Work out the finished part from the listing and answer in its coordinate system (mm). A direction names the side the tool comes from. Round coordinates to 2 decimals unless told otherwise and drop trailing zeros. Order: outer loops, then holes, each group sorted by start corner. A loop starts at its lowest first (then second) coordinate and runs counter-clockwise, first axis right, second up. Notation, with made-up numbers: (-36, -2.5) -> (-17, -2.5) arc R12 ccw to (-17, 3.5) -> close; hole circle Ø5 at (47.5, 52). An arc over 180 degrees is marked (long way). Use one line per item in the form item = value.
```python
from build123d import *

# Parameters (mm, degrees)
SKETCH_2_W          = 66
SKETCH_2_H          = 54
EXTRUDE_1_DEPTH     = 4
HOLE_WIZARD_M3_1_D  = 2.5
SKETCH_7_W          = 5
SKETCH_7_H          = 7.5
SKETCH_7_W_2        = 5.7
SKETCH_7_H_2        = 5.7
SKETCH_7_W_3        = 19
SKETCH_7_H_3        = 13
SKETCH_7_W_4        = 12
SKETCH_7_H_4        = 11.5
CUT_EXTRUDE_1_DEPTH = 4


with BuildPart() as part:
    # 草图2 → 凸台-拉伸1 (new body)
    with BuildSketch(Plane(origin=(0, 0, 0), x_dir=(1, 0, 0), z_dir=(0, 1, 0))):
        with Locations((33, -27)):
            Rectangle(SKETCH_2_W, SKETCH_2_H)
    extrude(amount=EXTRUDE_1_DEPTH)

    # M3 螺纹孔1 (through all)
    with Locations(Plane(origin=(0, 4, 0), x_dir=(1, 0, 0), z_dir=(0, 1, 0))):
        with Locations((3, -3), (3, -51), (63, -51), (63, -3)):
            Hole(HOLE_WIZARD_M3_1_D / 2)

    # 草图7 → 切除-拉伸1 (cut)
    with BuildSketch(Plane(origin=(0, 4, 0), x_dir=(1, 0, 0), z_dir=(0, 1, 0))):
        with Locations((24.815080673, -47.25)):
            Rectangle(SKETCH_7_W, SKETCH_7_H)
        with Locations((13.157222246, -9.084625301)):
            Rectangle(SKETCH_7_W_2, SKETCH_7_H_2)
        with Locations((13.157222246, -20.480710499)):
            Rectangle(SKETCH_7_W_2, SKETCH_7_H_2)
        with Locations((32.935955056, -12.734625301)):
            Rectangle(SKETCH_7_W_3, SKETCH_7_H_3)
        with Locations((43.342846772, -45.25)):
            Rectangle(SKETCH_7_W_4, SKETCH_7_H_4)
    extrude(amount=-CUT_EXTRUDE_1_DEPTH, mode=Mode.SUBTRACT)


solid = part.part
```
Item 1: A flat-ended cylindrical pin translates along its axis: P1, Ø3, axis at x = 34.5, z = 17, coming from the -Y side. Find the tip coordinate at first contact, or state that the pin passes through.
Findings:
P1 = through
Item 2: The part is cut by section A-A, the plane z = 8. Give the vertices of the cut face in (x, y), and give its area (3 significant figures).
Findings:
outline = (0, 0) -> (10.31, 0) -> (10.31, 4) -> (0, 4) -> close; (16.01, 0) -> (23.44, 0) -> (23.44, 4) -> (16.01, 4) -> close; (42.44, 0) -> (66, 0) -> (66, 4) -> (42.44, 4) -> close
area = 165 mm^2
Item 3: The part is cut by section D-D, the plane x = 28. Give the vertices of the cut face in (y, z), and give its area (3 significant figures).
Findings:
outline = (0, 0) -> (4, 0) -> (4, 6.23) -> (0, 6.23) -> close; (0, 19.23) -> (4, 19.23) -> (4, 54) -> (0, 54) -> close
area = 164 mm^2
Item 4: Determine the mould class of faces 3 (the flat face through (42.436, 2, 13)), 4 (the flat face through (33, 2, 54)), 5 (the flat face through (33, 4, 27)) for opening direction Z: released by +Z, released by -Z, zero draft, split by the parting line, or undercut.
Findings:
face_3 = undercut
face_4 = released by +Z
face_5 = zero draft
Item 5: Consider line 1 along X through (y, z) = (3.55, 47.5); line 2 along X through (y, z) = (1.5, 18.5); line 3 along Z through (x, y) = (15.5, 1.55). Determine where each line is inside the solid, lowest interval first.
Findings:
line_1 = 0 to 22.32, 27.32 to 37.34, 49.34 to 66
line_2 = 0 to 10.31, 16.01 to 23.44, 42.44 to 66
line_3 = 0 to 6.23, 11.93 to 17.63, 23.33 to 54
Item 6: The part is cut by section B-B, the plane y = 1.7. Give the number of separate pieces and of enclosed holes in the cut face, and give its area (3 significant figures).
Findings:
separate_pieces = 1
enclosed_holes = 9
area = 3,060 mm^2
Item 7: For faces 1 (the flat face through (0, 2, 27)), 2 (the flat face through (10.307, 2, 21)), determine the directions among +Z, -Z, +X, -X, +Y, -Y from which every point of the face is accessible in a straight line to the end or side of a thin tool.
Findings:
face_1 = +Z, -Z, -X, +Y, -Y
face_2 = +Y, -Y
Item 8: The part is cut by section C-C, the plane x = 63. Give the vertices of the cut face in (y, z).
Findings:
outline = (0, 0) -> (4, 0) -> (4, 1.75) -> (0, 1.75) -> close; (0, 4.25) -> (4, 4.25) -> (4, 49.75) -> (0, 49.75) -> close; (0, 52.25) -> (4, 52.25) -> (4, 54) -> (0, 54) -> close
